Geometry: final body of the model. Coordinates: model frame, mm. A direction names the side the tool comes from. Coordinates: 2 decimals unless noted, no trailing zeros. Write each loop counter-clockwise with the first axis right and the second up, starting at its lowest first coordinate (ties: lowest second). Pieces come first, ordered by that corner, then holes. Notation, with made-up numbers: (34.25, -10) -> (77.25, -10) arc R24 ccw to (77.25, 18) -> close; hole circle Ø3 at (-31.5, 27). An arc over 180 degrees is marked (long way). One line per item, written item: value.
```python
from build123d import *

# Parameters (mm, degrees)
BOSS_EXTRUDE1_DEPTH                                 = 13.865
BOSS_EXTRUDE1_DEPTH_BACK                            = 13.865
SKETCH1_R                                           = 2.75
SKETCH2_R                                           = 2.75
SKETCH2_R_2                                         = 2.25
CUT_EXTRUDE1_DEPTH                                  = 5
CUT_EXTRUDE2_START                                  = -5
SKETCH3_R                                           = 2.75
SKETCH3_R_2                                         = 2.25
CUT_EXTRUDE2_DEPTH                                  = 5
CSK_FOR_M3_COUNTERSUNK_FLAT_HEAD_SCREW1_D           = 3
CSK_FOR_M3_COUNTERSUNK_FLAT_HEAD_SCREW1_DEPTH       = 10
CSK_FOR_M3_COUNTERSUNK_FLAT_HEAD_SCREW1_CSINK_D     = 3.5
CSK_FOR_M3_COUNTERSUNK_FLAT_HEAD_SCREW1_CSINK_ANGLE = 90
CSK_FOR_M3_COUNTERSUNK_FLAT_HEAD_SCREW1_TIP         = 0.901290929
CSK_FOR_M3_COUNTERSUNK_FLAT_HEAD_SCREW2_D           = 3
CSK_FOR_M3_COUNTERSUNK_FLAT_HEAD_SCREW2_DEPTH       = 10
CSK_FOR_M3_COUNTERSUNK_FLAT_HEAD_SCREW2_CSINK_D     = 3.5
CSK_FOR_M3_COUNTERSUNK_FLAT_HEAD_SCREW2_CSINK_ANGLE = 90
CSK_FOR_M3_COUNTERSUNK_FLAT_HEAD_SCREW2_TIP         = 0.901290929
SKETCH8_W                                           = 7.4
SKETCH8_H                                           = 4
CUT_EXTRUDE3_DEPTH                                  = 3
SKETCH9_R                                           = 1.25
CUT_EXTRUDE4_DEPTH                                  = 16.023608921


with BuildPart() as part:
    # Sketch1 → Boss-Extrude1 (new, two sides: drawn at the far end of the back side and taken through both)
    with BuildSketch(Plane(origin=(0, 0, 0), x_dir=(0, 0, -1), z_dir=(1, 0, 0)).offset(-BOSS_EXTRUDE1_DEPTH_BACK)):
        Circle(SKETCH1_R)
    extrude(amount=BOSS_EXTRUDE1_DEPTH + BOSS_EXTRUDE1_DEPTH_BACK)

    # Sketch2 → Cut-Extrude1 (cut)
    with BuildSketch(Plane(origin=(13.865, 0, 0), x_dir=(0, 0, -1), z_dir=(1, 0, 0))):
        Circle(SKETCH2_R)
        Circle(SKETCH2_R_2, mode=Mode.SUBTRACT)
    extrude(amount=-CUT_EXTRUDE1_DEPTH, mode=Mode.SUBTRACT)

    # Sketch3 → Cut-Extrude2 (cut)
    with BuildSketch(Plane.ZY.offset(13.865).offset(CUT_EXTRUDE2_START)):
        with Locations(Location((0, 0, 0), (0, 0, 180))):
            Circle(SKETCH3_R)
        with Locations(Location((0, 0, 0), (0, 0, 180))):
            Circle(SKETCH3_R_2, mode=Mode.SUBTRACT)
    extrude(amount=CUT_EXTRUDE2_DEPTH, mode=Mode.SUBTRACT)

    # CSK for M3 Countersunk Flat Head Screw1
    with Locations(Plane.ZY.offset(13.865)):
        with Locations((0, 0)):
            CounterSinkHole(CSK_FOR_M3_COUNTERSUNK_FLAT_HEAD_SCREW1_D / 2, CSK_FOR_M3_COUNTERSUNK_FLAT_HEAD_SCREW1_CSINK_D / 2, depth=CSK_FOR_M3_COUNTERSUNK_FLAT_HEAD_SCREW1_DEPTH, counter_sink_angle=CSK_FOR_M3_COUNTERSUNK_FLAT_HEAD_SCREW1_CSINK_ANGLE)
            with Locations((0, 0, -(CSK_FOR_M3_COUNTERSUNK_FLAT_HEAD_SCREW1_DEPTH + CSK_FOR_M3_COUNTERSUNK_FLAT_HEAD_SCREW1_TIP / 2))):  # 118° drill point
                Cone(0, CSK_FOR_M3_COUNTERSUNK_FLAT_HEAD_SCREW1_D / 2, CSK_FOR_M3_COUNTERSUNK_FLAT_HEAD_SCREW1_TIP, mode=Mode.SUBTRACT)

    # CSK for M3 Countersunk Flat Head Screw2
    with Locations(Plane(origin=(13.865, 0, 0), x_dir=(0, 0, -1), z_dir=(1, 0, 0))):
        with Locations((0, 0)):
            CounterSinkHole(CSK_FOR_M3_COUNTERSUNK_FLAT_HEAD_SCREW2_D / 2, CSK_FOR_M3_COUNTERSUNK_FLAT_HEAD_SCREW2_CSINK_D / 2, depth=CSK_FOR_M3_COUNTERSUNK_FLAT_HEAD_SCREW2_DEPTH, counter_sink_angle=CSK_FOR_M3_COUNTERSUNK_FLAT_HEAD_SCREW2_CSINK_ANGLE)
            with Locations((0, 0, -(CSK_FOR_M3_COUNTERSUNK_FLAT_HEAD_SCREW2_DEPTH + CSK_FOR_M3_COUNTERSUNK_FLAT_HEAD_SCREW2_TIP / 2))):  # 118° drill point
                Cone(0, CSK_FOR_M3_COUNTERSUNK_FLAT_HEAD_SCREW2_D / 2, CSK_FOR_M3_COUNTERSUNK_FLAT_HEAD_SCREW2_TIP, mode=Mode.SUBTRACT)

    # Sketch8 → Cut-Extrude3 (cut)
    with BuildSketch(Plane.XY.offset(-5.34)):
        Rectangle(SKETCH8_W, SKETCH8_H)
    extrude(amount=CUT_EXTRUDE3_DEPTH, mode=Mode.SUBTRACT)

    # Sketch9 → Cut-Extrude4 (cut, through all)
    with BuildSketch(Plane(origin=(0, 0, -2.34), x_dir=(-1, 0, 0), z_dir=(0, 0, -1))):
        Circle(SKETCH9_R)
    extrude(amount=-CUT_EXTRUDE4_DEPTH, mode=Mode.SUBTRACT)


solid = part.part
```
(1) Section C-C (x = 8). Return the cut outline in (y, z), then the cut area to 3 significant figures.
Responses:
outline: circle Ø5.5 at (0, 0); hole circle Ø3 at (0, 0)
area: 16.7 mm2
(2) Section A-A (x = 0). Return the cut outline in (y, z).
Responses:
outline: (-1.44, -2.34) -> (-1.25, -2.34) -> (-1.25, 2.45) arc R2.75 ccw to start; (1.25, -2.34) -> (1.44, -2.34) arc R2.75 ccw to (1.25, 2.45) -> close
(3) Line query: line 1 (Y direction, x = -8.75, z = 0); line 2 (Y direction, x = 10.5, z = 0); line 3 (X direction, y = -1.65, z = -2.15) (3 decimals). Output: solid intervals per line, ascending. Write a range as [from, to].
Responses:
line 1: y = [-2.75, -1.5], [1.5, 2.75]
line 2: y = [-2.25, -1.5], [1.5, 2.25]
line 3: x = [-8.865, 8.865]
(4) First-contact query: pin 1 (3 mm diameter, centred on x = -10.5, y = 2, fed in from -Z); pin 2 (3 mm diameter, centred on x = -1.5, y = 0.5, fed in from -Z); pin 3 (2.5 mm diameter, centred on y = 0, z = 0, fed in from -X). Flat tips, straight axial feed; report the tip coordinate or a pass-through.
Responses:
pin 1: stops at z = -2.19
pin 2: stops at z = -2.34
pin 3: stops at x = -3.71
(5) Pull-direction query (Y, two-part tool) for faces 1 (the flat face through (13.865, -2, 0)), 2 (the conical face through (-3.12, -0.25, -0.06)), 3 (the cylindrical face through (11.4, 2.23, 0.29)); classes: released by +Y, released by -Y, zero draft, split by the parting line, or undercut.
Responses:
face 1: zero draft
face 2: undercut
face 3: split by the parting line
(6) Reachability of faces 4 (the cylindrical face through (8.67, 0.07, -1.5)), 5 (the cylindrical face through (-11.33, -1.52, 1.66)), 6 (the flat face through (-1, 1, -2.34)) from +Z, -Z, +X, -X, +Y, -Y: full face, straight path, thin tool, end or side. Return the list, or none.
Responses:
face 4: +X
face 5: -X
face 6: -Z, +Y, -Y
(7) Section B-B (x = 12.25). Return the cut outline in (y, z).
Responses:
outline: circle Ø4.5 at (0, 0); hole circle Ø3 at (0, 0)
